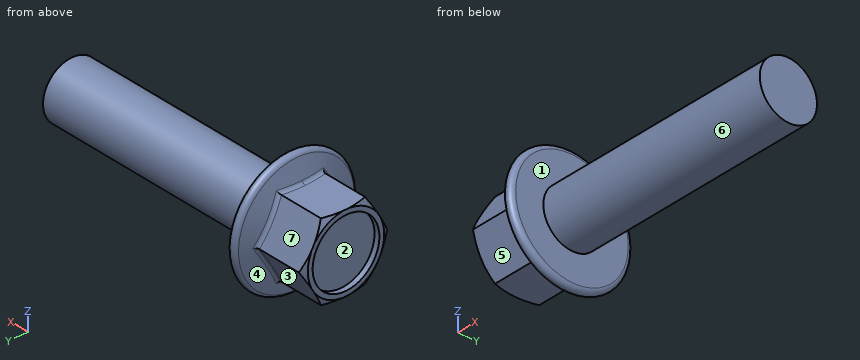
from build123d import *

# Parameters (mm, degrees)
SKETCH2_R         = 4.665127021
HEX_DIE_DEPTH     = 6.7
FLANGEHEXFILLET_R = 0.4
SKETCH4_R         = 3.5
INDENT_DEPTH      = 0.558333333


with BuildPart() as part:
    # BodySke → Base-Revolve (revolve)
    with BuildSketch(Plane.XY, mode=Mode.PRIVATE) as base_revolve_sk:
        Polygon((6.7, 3), (6.7, 4.618937644), (0.357343816, 4.618937644), (0, 4), (0, 0), (31.7, 0), (31.7, 3), align=None)
    revolve(base_revolve_sk.sketch.rotate(Axis((-25.4, 0, 0), (1, 0, 0)), 90), axis=Axis((-25.4, 0, 0), (1, 0, 0)))

    # Sketch2 → Hex-Die (cut)
    with BuildSketch(Plane(origin=(0, 0, 0), x_dir=(0, 0, -1), z_dir=(1, 0, 0))):
        Circle(SKETCH2_R)
        Polygon((-4, 2.309401087), (0, 4.618802174), (4, 2.309401087), (4, -2.309401087), (0, -4.618802174), (-4, -2.309401087), align=None, mode=Mode.SUBTRACT)
    extrude(amount=HEX_DIE_DEPTH, mode=Mode.SUBTRACT)

    # Sketch5 → Flange (revolve)
    with BuildSketch(Plane.XY, mode=Mode.PRIVATE) as flange_sk:
        with BuildLine():
            Line((3.520486732, 0), (5.73015369, 6.071010072))
            ThreePointArc((5.73015369, 6.071010072), (6.286824089, 6.392403877), (6.7, 5.9))
            Line((6.7, 5.9), (6.7, 0))
            Line((6.7, 0), (3.520486732, 0))
        make_face()
    revolve(flange_sk.sketch.rotate(Axis((0, 0, 0), (1, 0, 0)), 90), axis=Axis((0, 0, 0), (1, 0, 0)))

    # FlangeHexFillet
    flangehexfillet_edges = [part.edges().sort_by_distance(p)[0] for p in [
        (5.036325168, 1.159737723, 4),
        (4.976367673, 3.46410163, 2),
        (4.976367673, 3.46410163, -2),
        (4.976367669, 0, -4),
        (4.976367673, -3.46410163, -2),
        (4.976367673, -3.46410163, 2),
        (5.036325168, -1.159737723, 4),
    ]]
    fillet(flangehexfillet_edges, radius=FLANGEHEXFILLET_R)

    # Sketch4 → Indent (cut)
    with BuildSketch(Plane(origin=(0, 0, 0), x_dir=(0, 0, -1), z_dir=(1, 0, 0))):
        Circle(SKETCH4_R)
    extrude(amount=INDENT_DEPTH, mode=Mode.SUBTRACT)


solid = part.part
Read the model definition and answer for the solid it produces. Units are mm, in the model's axes. Face numbers are marked on the shaded views. A direction names the side the tool comes from. Coordinates: 2 decimals unless noted, no trailing zeros. Loops run counter-clockwise (first coordinate to the right, second up) from the corner with the lowest first, then second, coordinate; pieces in that order, holes last.
Q1. Each of these flat-tipped pins is pushed along its axis until it touches: pin 1 Ø1 at (x, z) = (7, 3) entering from -Y; pin 2 Ø5 at (x, y) = (3.5, -0.5) entering from -Z; pin 3 Ø4 at (x, z) = (23, -3) entering from +Y. Where does it stop, or does it pass through?
Q2. Which of the six approach directions +Z, -Z, +X, -X, +Y, -Y give full straight-line access (tool end or side, diameter ignored) to the marked faces 5, 6 and 7?
Q3. The mould has two halves that part along Z. Classify the marked faces 1, 2, 3 and 4: +Z half, -Z half, draft (parallel to the pull), parting line (faces both ways), or undercut.
Q4. The part is cut by section A-A on x = 23. Write down the section's boundary in (y, z).
Q5. Consider probe 1 along X at (y, z) = (-3, 0.5); probe 2 along Y at (x, z) = (0.25, 0); probe 3 along Y at (x, z) = (0.2, 0). Determine where each line is inside the solid, lowest interval first.
Results below:
1. pin 1: stops at y = -5.6
1. pin 2: stops at z = -6.35
1. pin 3: stops at y = 2.83
2. face 5: -Z, -X, -Y
2. face 6: +X
2. face 7: +Z, -X, +Y
3. face 1: draft
3. face 2: undercut
3. face 3: -Z half
3. face 4: parting line
4. outline: circle Ø6 at (0, 0)
5. probe 1: x = 0.56 to 6.7
5. probe 2: y = -4.43 to -3.5, 3.5 to 4.43
5. probe 3: y = -4.35 to -3.5, 3.5 to 4.35
